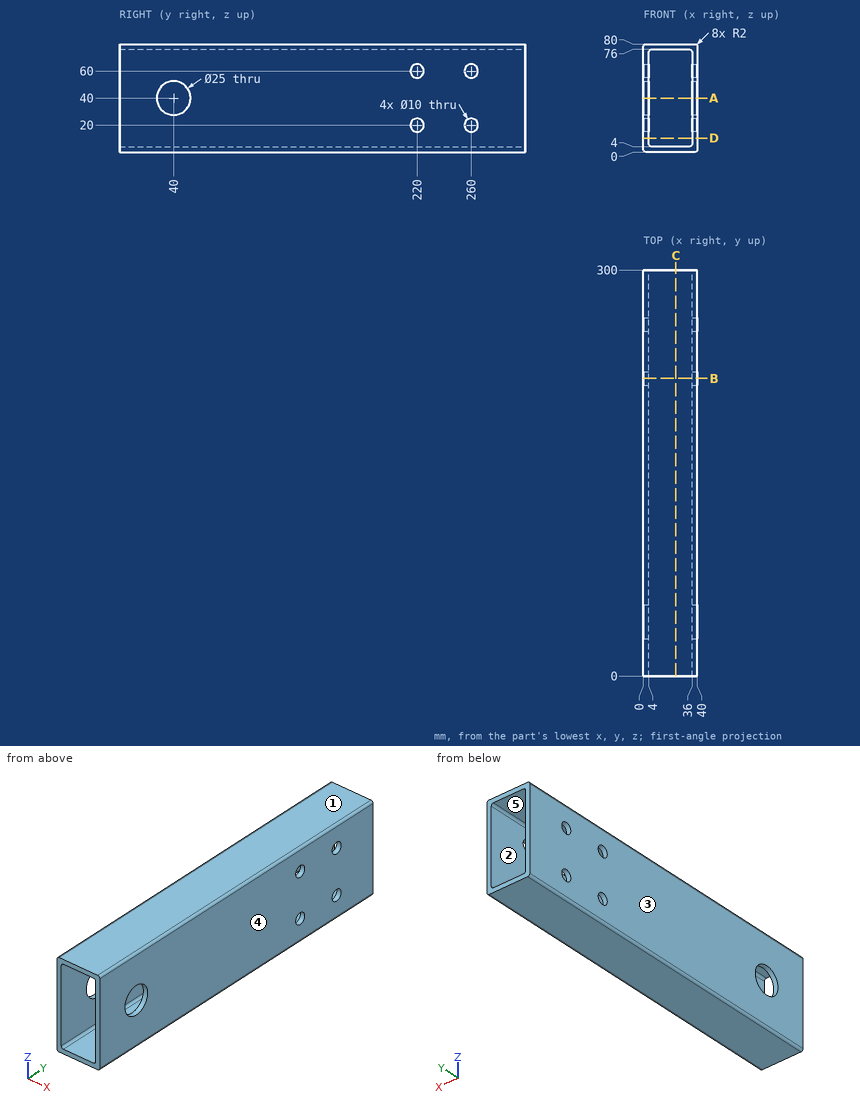
Print and shaded views of the part. All mm, measured from the part's lowest x, y and z. A direction names the side the tool comes from. Round coordinates to 2 decimals unless told otherwise and drop trailing zeros. Write each loop counter-clockwise with the first axis right and the second up, starting at its lowest first coordinate (ties: lowest second). Pieces come first, ordered by that corner, then holes. Notation, with made-up numbers: M 62,69 L 102,69 A31 cw 102,105 Z; hole C 16,-2 d6. An arc over 180 degrees is marked long. Use a Markdown table: item, result. Add a question column.
1. Slice it at C-C on x = 24. Give the cut face in (y, z), then the cut area to 3 significant figures.
2. Slice it at B-B on y = 220. Give the number of separate pieces and of enclosed holes in the cut face, then the cut area to 3 significant figures.
3. Slice it at D-D on z = 10.5. Give the cut face in (x, y), then the cut area to 3 significant figures.
4. Pull direction Z, two halves, no side cores. Call the marked faces 1, 2 and 3: released by +Z, released by -Z, zero draft, split by the parting line, or undercut.
5. Flat gauge pin, fed straight in: P1, Ø6, axis at y = 260, z = 20, coming from the -X side. Where does the tip first touch, or does it go through?
6. Drill centre lines: probe 1 along Y at (x, z) = (37, 60); probe 2 along Z at (x, y) = (37, 260); probe 3 along Z at (x, y) = (21.5, 231). Where is each one in solid material? Low to high.
7. Slice it at A-A on z = 40. Give the cut face in (x, y).
8. 3-axis set-ups, long thin cutter, end or side, ignore diameter. For the marked faces 4 and 5: which of +Z, -Z, +X, -X, +Y, -Y reach the whole face in a straight line?
Reply:
| question | item | result |
|---|---|---|
| 1 | outline | M 0,0 L 300,0 L 300,4 L 0,4 Z; M 0,76 L 300,76 L 300,80 L 0,80 Z |
| 1 | area | 2,400 mm^2 |
| 2 | separate pieces | 4 |
| 2 | enclosed holes | 0 |
| 2 | area | 736 mm^2 |
| 3 | outline | M 0,0 L 4,0 L 4,300 L 0,300 Z; M 36,0 L 40,0 L 40,300 L 36,300 Z |
| 3 | area | 2,400 mm^2 |
| 4 | face 1 | released by +Z |
| 4 | face 2 | undercut |
| 4 | face 3 | zero draft |
| 5 | P1 | passes through |
| 6 | probe 1 | y = 0 to 215, 225 to 255, 265 to 300 |
| 6 | probe 2 | z = 0 to 15, 25 to 55, 65 to 80 |
| 6 | probe 3 | z = 0 to 4, 76 to 80 |
| 7 | outline | M 0,0 L 4,0 L 4,27.5 L 0,27.5 Z; M 0,52.5 L 4,52.5 L 4,300 L 0,300 Z; M 36,0 L 40,0 L 40,27.5 L 36,27.5 Z; M 36,52.5 L 40,52.5 L 40,300 L 36,300 Z |
| 8 | face 4 | +Z, -Z, +X, +Y, -Y |
| 8 | face 5 | +Y, -Y |
